Here's how the part is built. I have some questions about the finished solid (model axes, mm). A direction names the side the tool comes from. Round coordinates to 2 decimals unless told otherwise and drop trailing zeros. Loops run counter-clockwise (first coordinate to the right, second up) from the corner with the lowest first, then second, coordinate; pieces in that order, holes last. Notation, with made-up numbers: (38, 74) -> (59, 74) arc R32 ccw to (59, 112) -> close; hole circle Ø9 at (-3.75, 17.5). An arc over 180 degrees is marked (long way). Use one line per item in the form item = value. Start each with the question number.
Item 1: If I drill on L1, parallel to X at y = -16.3, z = 0; L2, parallel to Y at x = 4.5, z = 12; L3, parallel to X at y = -12.25, z = -10, over which ranges is the centre line in solid material (lowest first)? Write a range as [from, to].
Item 2: For faces 5 (the face through (-12.932, -7.395, -5.362)), 6 (the face through (17, -10, 0)), which set-ups out of +Z, -Z, +X, -X, +Y, -Y let a thin tool reach every point of the face, with its end or its side?
Item 3: If we section it at B-B (x = -7): Write out the boundary of the cut face in (y, z), then the cut area to 3 significant figures.
Item 4: Thinking about a two-plate mould opening in Z: for faces 1 (the face through (10, -17.5, -3.2)), 2 (the face through (8, -10, -16)), 3 (the face through (11, -20, 0)), 4 (the face through (-5.1, -15, 9.4)), which applies, released by +Z, released by -Z, zero draft, split by the parting line, or undercut?
Item 5: I'm going to push flat-ended pins straight in: pin 1 Ø5 at (y, z) = (-6.5, 5) entering from -X; pin 2 Ø1.5 at (x, z) = (9, -6) entering from +Y. Where does each tip first touch, or does it pass through?
Item 6: If we section it at C-C (y = -9): Write out the boundary of the cut face in (x, z).
Item 7: If we section it at D-D (x = 11): Write out the boundary of the cut face in (y, z).
Item 8: If we section it at A-A (z = 0): Write out the boundary of the cut face in (x, y), then the cut area to 3 significant figures.
```python
from build123d import *

# Parameters (mm, degrees)
F0_R      = 16
F0_R_2    = 10.5
F1_DEPTH  = 20
F2_R      = 12.5
F3_DEPTH  = 15
F4_DEPTH  = 15.001
F5_R      = 14
F6_DEPTH  = 15
F8_W      = 20
F8_H      = 16
F9_DEPTH  = 2
F11_DEPTH = 20
F14_DEPTH = 20


with BuildPart() as f1:
    # F0 (on Front) → F1 (new body)
    with BuildSketch(Plane.XZ):
        Circle(F0_R)
        Circle(F0_R_2, mode=Mode.SUBTRACT)
    extrude(amount=F1_DEPTH)

    # F2 (on face) → F3 (join)
    with BuildSketch(Plane.XZ.offset(20)):
        Circle(F2_R)
    extrude(amount=-F3_DEPTH)

    # F4 (cut, through all): a face of the model
    f4_faces = [f1.faces().sort_by_distance(p)[0] for p in [
        (0, -5, 0),
    ]]
    extrude(f4_faces, amount=-F4_DEPTH, mode=Mode.SUBTRACT)

    # F5 (on face) → F6 (cut)
    with BuildSketch(Plane(origin=(0, 0, 0), x_dir=(-1, 0, 0), z_dir=(0, 1, 0))):
        Circle(F5_R)
    extrude(amount=-F6_DEPTH, mode=Mode.SUBTRACT)

    # F8 (on offset) → F9 (join)
    with BuildSketch(Plane.YZ.offset(15)):
        with Locations((-10, -8)):
            Rectangle(F8_W, F8_H)
        with Locations((-10, 8)):
            Rectangle(F8_W, F8_H)
    extrude(amount=F9_DEPTH)

    # F10 (on face) → F11 (join)
    with BuildSketch(Plane.XZ.offset(20)):
        with BuildLine():
            Line((15, 16), (0, 16))
            ThreePointArc((0, 16), (9.1355287257, 13.1355287257), (15, 5.5677643628))
            Line((15, 5.5677643628), (15, 16))
        make_face()
    extrude(amount=-F11_DEPTH)

    # F13 (on face) → F14 (join)
    with BuildSketch(Plane.XZ.offset(20)):
        with BuildLine():
            Line((0, -16), (15, -16))
            Line((15, -16), (15, -5.5677643628))
            ThreePointArc((15, -5.5677643628), (9.1355287257, -13.1355287257), (0, -16))
        make_face()
    extrude(amount=-F14_DEPTH)


solid = f1.part
```
Values found:
q1.L1 = [-16, -10.5], [10.5, 17]
q1.L2 = [-20, -15]
q1.L3 = [-12.49, -9.8], [9.8, 17]
q2.face_5 = +Y
q2.face_6 = +Z, -Z, +X, +Y, -Y
q3.outline = (-20, -14.39) -> (0, -14.39) -> (0, -12.12) -> (-15, -12.12) -> (-15, -7.83) -> (-20, -7.83) -> close; (-20, 7.83) -> (-15, 7.83) -> (-15, 12.12) -> (0, 12.12) -> (0, 14.39) -> (-20, 14.39) -> close
q3.area = 134 mm2
q4.face_1 = undercut
q4.face_2 = released by -Z
q4.face_3 = zero draft
q4.face_4 = undercut
q5.pin_1 = -15.8
q5.pin_2 = -15
q6.outline = (0, -16) -> (17, -16) -> (17, 16) -> (0, 16) arc R16 ccw to start; hole circle Ø28 at (0, 0)
q7.outline = (-20, -16) -> (0, -16) -> (0, -8.66) -> (-15, -8.66) -> (-15, 8.66) -> (0, 8.66) -> (0, 16) -> (-20, 16) -> close
q8.outline = (-16, -20) -> (-10.5, -20) -> (-10.5, -15) -> (-14, -15) -> (-14, 0) -> (-16, 0) -> close; (10.5, -20) -> (17, -20) -> (17, 0) -> (14, 0) -> (14, -15) -> (10.5, -15) -> close
q8.area = 135 mm2
